For this review, take the finished solid that the model builds, in its own axes (mm). A direction names the side the tool comes from. Give positions to 0.01 mm unless a question says otherwise; leave off trailing zeros. Order: outer loops, then holes, each group sorted by start corner. A loop starts at its lowest first (then second) coordinate and runs counter-clockwise, first axis right, second up. Notation, with made-up numbers: (26, 88.5) -> (30, 88.5) arc R16 ccw to (30, 111.5) -> close; hole circle Ø7 at (32.25, 19). An arc over 180 degrees is marked (long way). Return JSON: item names as keys, results as strings. Group by question number.
1) For faces 4 (the face through (49.2, -3.175, 2.6)), 5 (the face through (45.2, -14.1, 12.1)), list the 3-axis set-ups (+Z, -Z, +X, -X, +Y, -Y) from which the entire face can be reached by the end or side of a thin tool; tool diameter is ignored.
2) Add section B-B (x = 56.5). Give the boundary of the cut face in (y, z) (3 decimals), then the cut area to 3 significant figures.
3) Add section A-A (z = 7). Give the boundary of the cut face in (x, y) (3 decimals), then the cut area to 3 significant figures.
4) The part is to be moulded in two halves that separate along Z. For faces 1 (the face through (42.21, -1.61, 2.94)), 2 (the face through (-1, -25.4, 0)), 3 (the face through (-1, -13, 24.311)), say which applies: released by +Z, released by -Z, zero draft, split by the parting line, or undercut.
5) To check wall thickness, follow line 1 along X through (y, z) = (-6.5, 13); line 2 along X through (y, z) = (-6.25, 10). State the ranges of each line that lie inside material, in increasing order.
from build123d import *

# Parameters (mm, degrees)
F0_W     = 132.060304
F0_H     = 48.622414
F0_R     = 8.918459
F0_R_2   = 5.530692
F1_DEPTH = 25.4
F2_DEPTH = 3.175


with BuildPart() as f1:
    # F0 (on Front) → F1 (new body)
    with BuildSketch(Plane.XZ):
        Rectangle(F0_W, F0_H)
        with Locations((49.285725, 8.370818)):
            Circle(F0_R, mode=Mode.SUBTRACT)
        with Locations((49.285725, 8.370818)):
            Circle(F0_R)
        with Locations((49.285725, 8.370818)):
            Circle(F0_R_2, mode=Mode.SUBTRACT)
    extrude(amount=F1_DEPTH)

    # F0 (on Front) → F2 (cut, symmetric)
    with BuildSketch(Plane.XZ):
        with Locations((49.285725, 8.370818)):
            Circle(F0_R)
        with Locations((49.285725, 8.370818)):
            Circle(F0_R_2, mode=Mode.SUBTRACT)
    extrude(amount=F2_DEPTH, both=True, mode=Mode.SUBTRACT)


solid = f1.part
Evaluation:
{
 "1": {"face 4": "+Y", "face 5": "+Y, -Y"},
 "2": {"outline": "(-25.4, -24.311) -> (0, -24.311) -> (0, 3.127) -> (-3.175, 3.127) -> (-3.175, 13.614) -> (0, 13.614) -> (0, 24.311) -> (-25.4, 24.311) -> close", "area": "1,200 mm^2"},
 "3": {"outline": "(-66.03, -25.4) -> (43.928, -25.4) -> (43.928, -3.175) -> (40.473, -3.175) -> (40.473, 0) -> (-66.03, 0) -> close; (54.644, -25.4) -> (66.03, -25.4) -> (66.03, 0) -> (58.098, 0) -> (58.098, -3.175) -> (54.644, -3.175) -> close", "area": "3,060 mm^2"},
 "4": {"face 1": "undercut", "face 2": "zero draft", "face 3": "released by +Z"},
 "5": {"line 1": "-66.03 to 46.26, 52.31 to 66.03", "line 2": "-66.03 to 44, 54.57 to 66.03"}
}
